Autodesk Inventor part; units mm, degrees
ref_plane "YZ Plane" through (0, 0, 0) normal (1, 0, 0) x (0, 1, 0)
ref_plane "XZ Plane" through (0, 0, 0) normal (0, 1, 0) x (-1, 0, 0)
ref_plane "XY Plane" through (0, 0, 0) normal (0, 0, 1) x (1, 0, 0)
sketch "Sketch1" plane through (0, 0, 0) normal (0, 0, 1) x (1, 0, 0)
  line L0 (-20, -20) -> (20, -20)
  line L1 (20, -20) -> (20, 20)
  line L2 (20, 20) -> (-20, 20)
  line L3 (-20, 20) -> (-20, -20)
  line L4 (-20, -20) -> (20, 20) construction
  line L5 (20, -20) -> (-20, 20) construction
  point P0 (0, 0)
  dimension "d0" = 40
  dimension "d1" = 40
extrude "Extrusion1" add sketch "Sketch1" along normal mid plane 1
sketch "Sketch2" plane through (0, 0, 0.5) normal (0, 0, 1) x (1, 0, 0)
  circle A0 centre (-17, 16) radius 2
  circle A1 centre (-17, 0) radius 2
  circle A2 centre (-17, -16) radius 2
  circle A3 centre (17, 16) radius 2
  circle A4 centre (17, 0) radius 2
  circle A5 centre (17, -16) radius 2
  line L0 (-20, 20) -> (-20, -20)
  point P0 (0, 0)
  dimension "d4" = 3
  dimension "d5" = 34
  dimension "d6" = 4
  dimension "d7" = 4
  dimension "d8" = 4
  dimension "d9" = 16
  dimension "d10" = 32
extrude "Extrusion2" cut sketch "Sketch2" against normal up to surface (1 mm away)
equation "\"d7\" = d6"
equation "\"d8\" = d6"
equation "\"d9\" = 0.5 * d10"
properties part number "26A" material "Gold"
Read the model definition and answer for the solid it produces. Units are mm, in the model's axes. Coordinates: 2 decimals unless noted, no trailing zeros. Loops run counter-clockwise (first coordinate to the right, second up) from the corner with the lowest first, then second, coordinate; pieces in that order, holes last. Notation, with made-up numbers: (-8, 76) -> (17, 76) arc R6 cw to (17, 80) -> close; hole circle Ø5 at (89, 42.5). An arc over 180 degrees is marked (long way). Return JSON: item names as keys, results as strings.
Item 1: Find section B-B (y = 16). Determine the outline of the cut face in (x, z), plus the area to 3 significant figures.
Answers:
{"outline": "(-20, -0.5) -> (-19, -0.5) -> (-19, 0.5) -> (-20, 0.5) -> close; (-15, -0.5) -> (15, -0.5) -> (15, 0.5) -> (-15, 0.5) -> close; (19, -0.5) -> (20, -0.5) -> (20, 0.5) -> (19, 0.5) -> close", "area": "32.0 mm2"}
Item 2: Find section C-C (z = -0.1). Determine the outline of the cut face in (x, y).
Answers:
{"outline": "(-20, -20) -> (20, -20) -> (20, 20) -> (-20, 20) -> close; hole circle Ø4 at (-17, -16); hole circle Ø4 at (-17, 0); hole circle Ø4 at (-17, 16); hole circle Ø4 at (17, -16); hole circle Ø4 at (17, 0); hole circle Ø4 at (17, 16)"}
Item 3: For a pull along Y with two mould halves and no side action, classify faces 1 (the flat face through (20, 0, 0)), 2 (the cylindrical face through (-17, -14, 0)), 3 (the flat face through (0, 20, 0)) as +Y half, -Y half, draft (parallel to the pull), parting line (faces both ways), or undercut.
Answers:
{"face 1": "draft", "face 2": "undercut", "face 3": "+Y half"}
Item 4: Find section A-A (x = 17). Determine the outline of the cut face in (y, z), plus the area to 3 significant figures.
Answers:
{"outline": "(-20, -0.5) -> (-18, -0.5) -> (-18, 0.5) -> (-20, 0.5) -> close; (-14, -0.5) -> (-2, -0.5) -> (-2, 0.5) -> (-14, 0.5) -> close; (2, -0.5) -> (14, -0.5) -> (14, 0.5) -> (2, 0.5) -> close; (18, -0.5) -> (20, -0.5) -> (20, 0.5) -> (18, 0.5) -> close", "area": "28.0 mm2"}
Item 5: Find the intervals of material crossed by probe 1 along Y at (x, z) = (17, 0); probe 2 along Y at (x, z) = (17.5, 0.4); probe 3 along X at (y, z) = (-0.5, 0.4), in increasing order.
Answers:
{"probe 1": "y = -20 to -18, -14 to -2, 2 to 14, 18 to 20", "probe 2": "y = -20 to -17.94, -14.06 to -1.94, 1.94 to 14.06, 17.94 to 20", "probe 3": "x = -20 to -18.94, -15.06 to 15.06, 18.94 to 20"}
Item 6: Find section D-D (x = -15.5). Determine the outline of the cut face in (y, z).
Answers:
{"outline": "(-20, -0.5) -> (-17.32, -0.5) -> (-17.32, 0.5) -> (-20, 0.5) -> close; (-14.68, -0.5) -> (-1.32, -0.5) -> (-1.32, 0.5) -> (-14.68, 0.5) -> close; (1.32, -0.5) -> (14.68, -0.5) -> (14.68, 0.5) -> (1.32, 0.5) -> close; (17.32, -0.5) -> (20, -0.5) -> (20, 0.5) -> (17.32, 0.5) -> close"}
